Answer from the drawing. Dimensions are ordinates in mm from the lowest x, y and z of the part. Round coordinates to 2 decimals unless told otherwise and drop trailing zeros. Write each loop counter-clockwise with the first axis right and the second up, starting at its lowest first coordinate (ties: lowest second). Pieces come first, ordered by that corner, then holes. Notation, with made-up numbers: (65, 37) - (91, 37) arc R13 ccw to (91, 57) - close; hole circle Ø10 at (-37, 25.25). An arc over 180 degrees is marked (long way). Return JSON: item names as keys, results as strings. Group by question number.
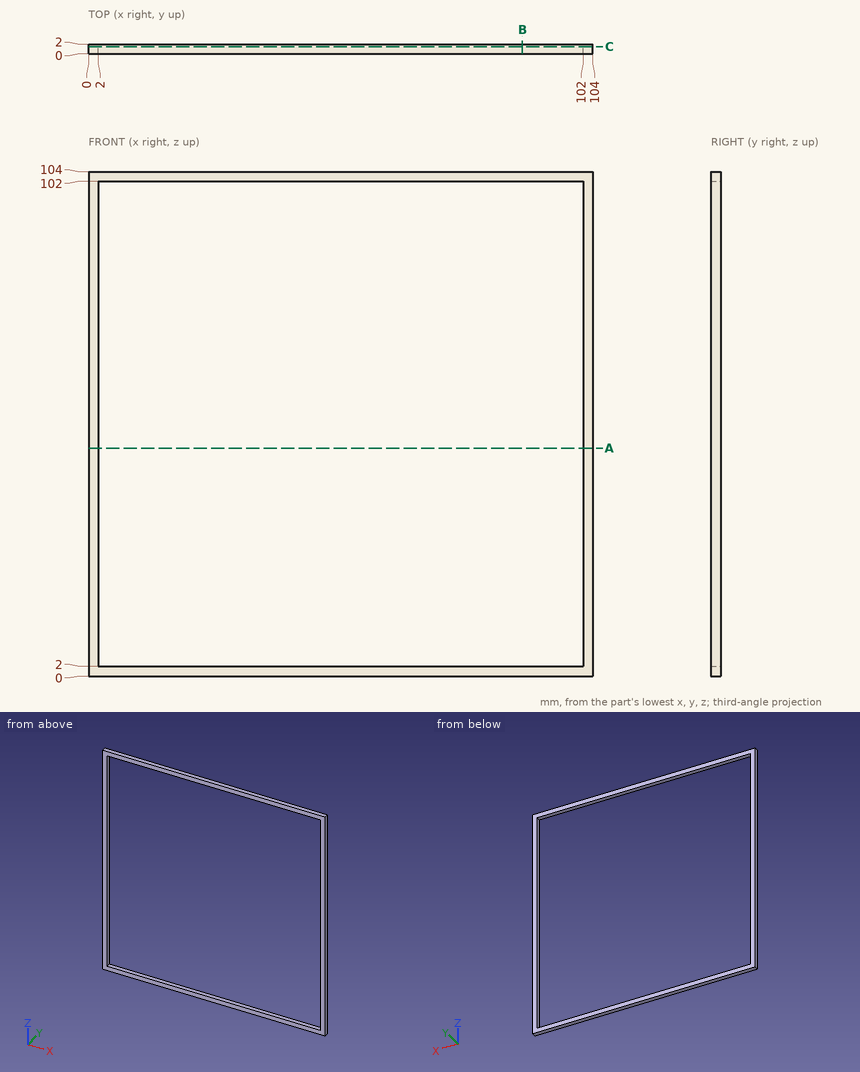
(1) Find section C-C (y = 1.45). Write down the section's boundary in (x, z), plus the area to 3 significant figures.
(2) Find section A-A (z = 47). Write down the section's boundary in (x, y), plus the area to 3 significant figures.
(3) Find section B-B (x = 89.5). Write down the section's boundary in (y, z), plus the area to 3 significant figures.
(4) Consider line 1 (X direction, y = 1.25, z = 33). Determine where the line is inside the solid, lowest interval first.
(5) A flat-ended cylindrical pin translates along its axis: pin 1 (1 mm diameter, centred on x = 61.5, y = 1.5, fed in from -Z). Find the tip coordinate at first contact, or state that the pin passes through.
Check sheet entries:
{
 "1": {"outline": "(0, 0) - (104, 0) - (104, 104) - (0, 104) - close; hole (2, 2) - (102, 2) - (102, 102) - (2, 102) - close", "area": "816 mm^2"},
 "2": {"outline": "(0, 0) - (2, 0) - (2, 2) - (0, 2) - close; (102, 0) - (104, 0) - (104, 2) - (102, 2) - close", "area": "8.00 mm^2"},
 "3": {"outline": "(0, 0) - (2, 0) - (2, 2) - (0, 2) - close; (0, 102) - (2, 102) - (2, 104) - (0, 104) - close", "area": "8.00 mm^2"},
 "4": {"line 1": "x = 0 to 2, 102 to 104"},
 "5": {"pin 1": "stops at z = 0"}
}
